Could you check a few things on this drawing? It's one solid part, dimensions in mm from its lowest x, y, z. A direction names the side the tool comes from. Give positions to 0.01 mm unless a question says otherwise; leave off trailing zeros. Loops run counter-clockwise (first coordinate to the right, second up) from the corner with the lowest first, then second, coordinate; pieces in that order, holes last.
1. Imagine slicing it at B-B (z = 7). List the corners of the cut face in (x, y) for me, plus the area to 3 significant figures.
2. Imagine slicing it at C-C (y = 81). List the corners of the cut face in (x, z) for me, plus the area to 3 significant figures.
3. For the marked faces 1 and 2, which set-ups out of +Z, -Z, +X, -X, +Y, -Y let a thin tool reach every point of the face, with its end or its side?
4. Imagine slicing it at A-A (x = 111). List the corners of the cut face in (y, z) for me.
5. For P1, Ø6.5, axis at x = 188.5, z = 22, coming from the +Y side; P2, Ø8, axis at x = 246, y = 66, coming from the +Z side; P3, Ø12, axis at x = 73.5, z = 4.5, coming from the -Y side; P4, Ø10, axis at y = 80, z = 19, coming from the +X side, each with a flat end and sliding along its axis, tell me the tip position at first contact or that it passes through.
6. I need wall thicknesses on line 1 along Z through (x, y) = (121, 77.5); line 2 along Z through (x, y) = (273, 23); line 3 along Y through (x, z) = (317, 7). Which ranges of each line are inside material? Lowest first, please.
7. Imagine slicing it at D-D (x = 265). List the corners of the cut face in (y, z) for me.
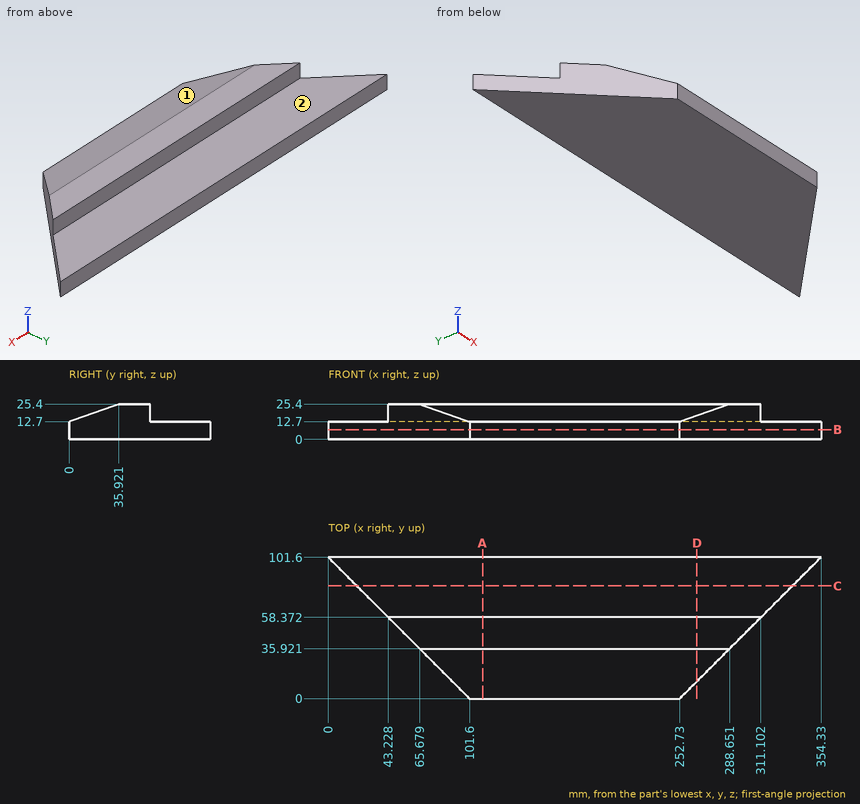
Derived:
1. outline: (0, 101.6) - (101.6, 0) - (252.73, 0) - (354.33, 101.6) - close
1. area: 25,700 mm2
2. outline: (20.6, 0) - (333.73, 0) - (333.73, 12.7) - (20.6, 12.7) - close
2. area: 3,980 mm2
3. face 1: +Z, +X, -X, -Y
3. face 2: +Z, +X, -X, +Y
4. outline: (0, 0) - (101.6, 0) - (101.6, 12.7) - (58.37, 12.7) - (58.37, 25.4) - (35.92, 25.4) - (0, 12.7) - close
5. P1: stops at y = 58.37
5. P2: stops at z = 12.7
5. P3: stops at y = 22.1
5. P4: passes through
6. line 1: z = 0 to 12.7
6. line 2: z = 0 to 20.83
6. line 3: y = 64.27 to 101.6
7. outline: (12.27, 0) - (101.6, 0) - (101.6, 12.7) - (58.37, 12.7) - (58.37, 25.4) - (35.92, 25.4) - (12.27, 17.04) - close
